from build123d import *

# Parameters (mm, degrees)
F1_DEPTH = 41.91
F3_D     = 6.7564
F5_D     = 6.7564
F5_DEPTH = 12.7
F5_TIP   = 2.0298273432
F7_D     = 6.7564
F8_R     = 3.4841261701
F9_DEPTH = 9.398


with BuildPart() as f1:
    # F0 (on Right) → F1 (new body)
    with BuildSketch(Plane.YZ):
        with BuildLine():
            add(Edge.make_bspline(
                [(-61.1524246633, 0), (-45.2024810028, 7.122572143), (-10.9378282084, 22.4237209544), (34.9882428649, 19.9241960467), (59.5360659063, 18.5881815851)],
                knots=[0, 0, 0, 0, 0.4654926392, 1, 1, 1, 1], degree=3))
            Line((-61.1524246633, 0), (59.5360659063, 0))
            Line((59.5360659063, 0), (59.5360659063, 18.5881815851))
        make_face()
    extrude(amount=F1_DEPTH)

    # F3 (through all)
    with Locations(Plane.YZ.offset(41.91)):
        with Locations((-22.8984840214, 4.5796968043), (42.2948487103, 4.5796968043)):
            Hole(F3_D / 2)

    # F5
    with Locations(Plane(origin=(0, 59.5360659063, 0), x_dir=(-1, 0, 0), z_dir=(0, 1, 0))):
        with Locations((-20.955, 12.6615148038)):
            Hole(F5_D / 2, depth=F5_DEPTH)
            with Locations((0, 0, -(F5_DEPTH + F5_TIP / 2))):  # 118° drill point
                Cone(0, F5_D / 2, F5_TIP, mode=Mode.SUBTRACT)

    # F7 (through all)
    with Locations(Plane(origin=(0, 0, 0), x_dir=(1, 0, 0), z_dir=(0, 0, -1))):
        with Locations((20.955, -50.1895733178)):
            Hole(F7_D / 2)

    # F8 (on face) → F9 (join)
    with BuildSketch(Plane(origin=(0, 0, 0), x_dir=(1, 0, 0), z_dir=(0, 0, -1))):
        with Locations((20.955, -50.1895733178)):
            Circle(F8_R)
    extrude(amount=-F9_DEPTH)


solid = f1.part
The model under review builds one solid part; all positions refer to its coordinate system, in mm. A direction names the side the tool comes from. Round coordinates to 2 decimals unless told otherwise and drop trailing zeros. Use CSV: the item, a comma, the result in double quotes.
(1) Clearance check with flat-ended pins moving along their axes: P1, Ø4, axis at y = -22.9, z = 4.58, coming from the +X side; P2, Ø3.5, axis at x = 21, y = 50.5, coming from the +Z side; P3, Ø10, axis at x = 9.5, y = 33, coming from the +Z side. State where each tip first meets the part, or that it passes through.
Working result:
P1,"passes through"
P2,"stops at z = 9.4"
P3,"stops at z = 19.91"
(2) Take a section at A-A, the plane z = 6.75. State how many separate pieces and enclosed holes the cut face has, plus the area to 3 significant figures.
Working result:
separate pieces,"3"
enclosed holes,"0"
area,"3,970 mm^2"
(3) The part is to be moulded in two halves that separate along Y. For faces 1 (the flat face through (0, 13, 9)), 2 (the cylindrical face through (23.445, 47.906, 16.737)), 3 (the conical face through (21.39, 45.16, 13.06)), 4 (the cylindrical face through (20.66, 45.67, 4.73)), say which applies: pulls with the +Y half, pulls with the -Y half, needs draft (parallel to the pull), parting line crosses it, or undercut.
Working result:
face 1,"needs draft"
face 2,"undercut"
face 3,"pulls with the +Y half"
face 4,"undercut"
(4) Machinability: for faces 5 (the cylindrical face through (17.59, 47.74, 12.96)), 6 (the flat face through (21, -2, 0)), 7 (the cylindrical face through (24.333, 50.128, 10.327)), which of the approach directions +Z, -Z, +X, -X, +Y, -Y give a long, thin tool a straight path to every point of the face, cutting with its end or side? Answer none if there is none.
Working result:
face 5,"+Y"
face 6,"-Z, +X, -X, +Y, -Y"
face 7,"+Z"
(5) For line 1 (Y direction, x = 21.5, z = 5); line 2 (Y direction, x = 26, z = 5.5); line 3 (Z direction, x = 3.5, y = -25), list the stretches that pass through material, from the lowest coordinate up.
Working result:
line 1,"y = -49.81 to -26.25, -19.55 to 38.94, 45.65 to 59.54"
line 2,"y = -48.64 to -26.15, -19.65 to 39.04, 45.55 to 59.54"
line 3,"z = 0 to 1.93, 7.22 to 14.17"
